Check sheet for the modelled part. Datum: model origin and axes. Units: mm. A direction names the side the tool comes from. Give positions to 0.01 mm unless a question says otherwise; leave off trailing zeros. Order: outer loops, then holes, each group sorted by start corner. A loop starts at its lowest first (then second) coordinate and runs counter-clockwise, first axis right, second up. Notation, with made-up numbers: (80.5, 48.5) - (126.5, 48.5) arc R30 cw to (126.5, 87.5) - close; hole circle Ø9 at (41, 56). An arc over 180 degrees is marked (long way). Answer in a Markdown table with one row per item.
from build123d import *

# Parameters (mm, degrees)
F0_W      = 620
F0_H      = 415
F1_DEPTH  = 5
F2_W      = 620
F2_H      = 5
F3_DEPTH  = 175
F5_D      = 5
F7_D      = 5
F9_D      = 5
F11_D     = 5
F13_D     = 5
F15_D     = 5
F17_D     = 5
F19_D     = 5
F19_DEPTH = 11
F20_W     = 620
F20_H     = 5
F21_DEPTH = 410
F23_D     = 5


with BuildPart() as f1:
    # F0 (on Top) → F1 (new body)
    with BuildSketch(Plane.XY):
        Rectangle(F0_W, F0_H)
    extrude(amount=F1_DEPTH)

    # F2 (on face) → F3 (join)
    with BuildSketch(Plane.XY.offset(5)):
        with Locations((0, -205)):
            Rectangle(F2_W, F2_H)
    extrude(amount=F3_DEPTH)

    # F5 (through all)
    with Locations(Plane.XZ.offset(207.5)):
        with Locations((300, 170)):
            Hole(F5_D / 2)

    # F7 (through all)
    with Locations(Plane.XZ.offset(207.5)):
        with Locations((300, 150)):
            Hole(F7_D / 2)

    # F9 (through all)
    with Locations(Plane.XZ.offset(207.5)):
        with Locations((-280, 170)):
            Hole(F9_D / 2)

    # F11 (through all)
    with Locations(Plane.XZ.offset(207.5)):
        with Locations((-280, 150)):
            Hole(F11_D / 2)

    # F13 (through all)
    with Locations(Plane.XZ.offset(207.5)):
        with Locations((-305, 10)):
            Hole(F13_D / 2)

    # F15 (through all)
    with Locations(Plane(origin=(0, 0, 0), x_dir=(1, 0, 0), z_dir=(0, 0, -1))):
        with Locations((290, 195)):
            Hole(F15_D / 2)

    # F17 (through all)
    with Locations(Plane(origin=(0, 0, 0), x_dir=(1, 0, 0), z_dir=(0, 0, -1))):
        with Locations((-290, 195)):
            Hole(F17_D / 2)

    # F19
    with Locations(Plane.XZ.offset(207.5)):
        with Locations((285, 25)):
            Hole(F19_D / 2, depth=F19_DEPTH)

    # F20 (on face) → F21 (join)
    with BuildSketch(Plane(origin=(0, -202.5, 0), x_dir=(-1, 0, 0), z_dir=(0, 1, 0))):
        with Locations((0, 177.5)):
            Rectangle(F20_W, F20_H)
    extrude(amount=F21_DEPTH)

    # F23 (through all)
    with Locations(Plane.XY.offset(180)):
        with Locations((-300, 197.5)):
            Hole(F23_D / 2)


solid = f1.part
(1) Cross-section at C-C, the plane z = 41. Record the cut outline in (x, y), then the cut area to 3 significant figures.
Geometry says:
| item | result |
|---|---|
| outline | (-310, -207.5) - (310, -207.5) - (310, -202.5) - (-310, -202.5) - close |
| area | 3,100 mm² |
(2) Gauge pin test, flat ends, axial feed: P1, Ø10, axis at x = 189, z = 58.5, coming from the +Y side; P2, Ø3, axis at x = 290, y = -195, coming from the -Z side. Record the tip position at first contact, or that the pin passes through.
Geometry says:
| item | result |
|---|---|
| P1 | y = -202.5 |
| P2 | z = 175 |
(3) Cross-section at B-B, the plane x = -76. Record the cut outline in (y, z), then the cut area to 3 significant figures.
Geometry says:
| item | result |
|---|---|
| outline | (-207.5, 0) - (207.5, 0) - (207.5, 5) - (-202.5, 5) - (-202.5, 175) - (207.5, 175) - (207.5, 180) - (-207.5, 180) - close |
| area | 5,000 mm² |
(4) Cross-section at A-A, the plane y = -38. Record the cut outline in (x, z).
Geometry says:
| item | result |
|---|---|
| outline | (-310, 0) - (310, 0) - (310, 5) - (-310, 5) - close; (-310, 175) - (310, 175) - (310, 180) - (-310, 180) - close |
(5) Mould release check, pull along Z, two halves, no side actions. Record for faces 3 (the flat face through (4, -3, 180)), 4 (the flat face through (-4, -202.5, 89)), 5 (the flat face through (-310, -1, 176)): pulls with the +Z half, pulls with the -Z half, needs draft (parallel to the pull), parting line crosses it, or undercut.
Geometry says:
| item | result |
|---|---|
| face 3 | pulls with the +Z half |
| face 4 | undercut |
| face 5 | needs draft |
(6) Thickness scan on L1, parallel to X at y = -205.1, z = 170; L2, parallel to Z at x = -20, y = 136; L3, parallel to X at y = 197, z = 178. Record the ranges inside material, lowest first.
Geometry says:
| item | result |
|---|---|
| L1 | -310 to -282.5, -277.5 to 297.5, 302.5 to 310 |
| L2 | 0 to 5, 175 to 180 |
| L3 | -310 to -302.45, -297.55 to 310 |
(7) Access from +Z, -Z, +X, -X, +Y, -Y to the whole of each face (thin tool, end or side, straight path). Record for faces 1 (the flat face through (-4, 5, 5)), 2 (the flat face through (310, -1, 176)).
Geometry says:
| item | result |
|---|---|
| face 1 | +X, -X, +Y |
| face 2 | +Z, -Z, +X, +Y, -Y |
